```python
from build123d import *

# Parameters (mm, degrees)
BOSS_EXTRUDE1_DEPTH     = 4
CUT_EXTRUDE1_DEPTH      = 8.549834435
CUT_EXTRUDE1_DEPTH_BACK = 8.549834435
FILLET1_R               = 0.5
SKETCH4_R               = 1.5
BOSS_EXTRUDE2_DEPTH     = 1
SKETCH5_R               = 3.2
BOSS_EXTRUDE3_DEPTH     = 2.5
FILLET2_R               = 1
SKETCH6_W               = 1
SKETCH6_H               = 4.4
SKETCH6_W_2             = 4.4
SKETCH6_H_2             = 1
CUT_EXTRUDE_THIN1_DEPTH = 1.25
SKETCH8_W               = 7.4
SKETCH8_H               = 7.4
BOSS_EXTRUDE4_DEPTH     = 1


with BuildPart() as part:
    # Sketch1 → Boss-Extrude1 (new, symmetric)
    with BuildSketch(Plane.XY):
        with BuildLine():
            Line((-1.75, 1), (-1.75, -4.5))
            ThreePointArc((-1.75, -4.5), (-2.5, -5), (-3.25, -4.5))
            Line((-3.25, -4.5), (-3.25, 0))
            Line((-3.25, 0), (-4, 0))
            Line((-4, 0), (-4, 2.9))
            ThreePointArc((-4, 2.9), (-3.853553391, 3.253553391), (-3.5, 3.4))
            Line((-3.5, 3.4), (3.5, 3.4))
            ThreePointArc((3.5, 3.4), (3.853553391, 3.253553391), (4, 2.9))
            Line((4, 2.9), (4, 0))
            Line((4, 0), (3.25, 0))
            Line((3.25, 0), (3.25, -4.5))
            ThreePointArc((3.25, -4.5), (2.5, -5), (1.75, -4.5))
            Line((1.75, -4.5), (1.75, 1))
            Line((1.75, 1), (-1.75, 1))
        make_face()
    extrude(amount=BOSS_EXTRUDE1_DEPTH, both=True)

    # Sketch3 → Cut-Extrude1 (cut, two sides: drawn at the far end of the back side and taken through both)
    with BuildSketch(Plane(origin=(0, 0, 0), x_dir=(0, 0, -1), z_dir=(1, 0, 0)).offset(-CUT_EXTRUDE1_DEPTH_BACK)):
        with BuildLine():
            Line((-3.2, -5), (-3.2, 2.1))
            ThreePointArc((-3.2, 2.1), (-3.053553391, 2.453553391), (-2.7, 2.6))
            Line((-2.7, 2.6), (2.7, 2.6))
            ThreePointArc((2.7, 2.6), (3.053553391, 2.453553391), (3.2, 2.1))
            Line((3.2, 2.1), (3.2, -5))
            Line((3.2, -5), (-3.2, -5))
        make_face()
    extrude(amount=CUT_EXTRUDE1_DEPTH + CUT_EXTRUDE1_DEPTH_BACK, mode=Mode.SUBTRACT)

    # Fillet1
    # the kernel refuses this fillet: 0.5 mm, written as the material it takes off along each edge
    with BuildSketch(Plane(origin=(-4.75, 3.4, -4), x_dir=(0, -1, 0), z_dir=(1, 0, 0))) as fillet1_piece_1:
        with BuildLine():
            CenterArc((FILLET1_R, -FILLET1_R), FILLET1_R, 90, 90)
            Line((0, -FILLET1_R), (0, 0))
            Line((0, 0), (FILLET1_R, 0))
        make_face()
    extrude(amount=9.5, mode=Mode.SUBTRACT)
    with BuildSketch(Plane(origin=(-4.75, 3.4, 4), x_dir=(0, -1, 0), z_dir=(1, 0, 0))) as fillet1_piece_2:
        with BuildLine():
            CenterArc((FILLET1_R, FILLET1_R), FILLET1_R, 180, 90)
            Line((0, FILLET1_R), (0, 0))
            Line((0, 0), (FILLET1_R, 0))
        make_face()
    extrude(amount=9.5, mode=Mode.SUBTRACT)

    # Sketch4 → Boss-Extrude2 (add)
    with BuildSketch(Plane(origin=(0, 3.4, 0), x_dir=(1, 0, 0), z_dir=(0, 1, 0))):
        with Locations(Location((0, 0, 0), (0, 0, 90))):
            Circle(SKETCH4_R)
    extrude(amount=BOSS_EXTRUDE2_DEPTH)

    # Sketch5 → Boss-Extrude3 (add)
    with BuildSketch(Plane(origin=(0, 4.4, 0), x_dir=(1, 0, 0), z_dir=(0, 1, 0))):
        with Locations(Location((0, 0, 0), (0, 0, 270))):
            Circle(SKETCH5_R)
    extrude(amount=BOSS_EXTRUDE3_DEPTH)

    # Fillet2
    fillet2_edges = [part.edges().sort_by_distance(p)[0] for p in [
        (0, 4.4, -3.2),
        (0, 6.9, -3.2),
    ]]
    fillet(fillet2_edges, radius=FILLET2_R)

    # Sketch6 → Cut-Extrude-Thin1 (cut)
    with BuildSketch(Plane(origin=(0, 6.9, 0), x_dir=(1, 0, 0), z_dir=(0, 1, 0))):
        Rectangle(SKETCH6_W, SKETCH6_H)
        Rectangle(SKETCH6_W_2, SKETCH6_H_2)
    extrude(amount=-CUT_EXTRUDE_THIN1_DEPTH, mode=Mode.SUBTRACT)

    # Sketch8 → Boss-Extrude4 (add)
    with BuildSketch(Plane(origin=(0, 3.4, 0), x_dir=(1, 0, 0), z_dir=(0, 1, 0))):
        Rectangle(SKETCH8_W, SKETCH8_H)
    extrude(amount=BOSS_EXTRUDE4_DEPTH)


solid = part.part
```
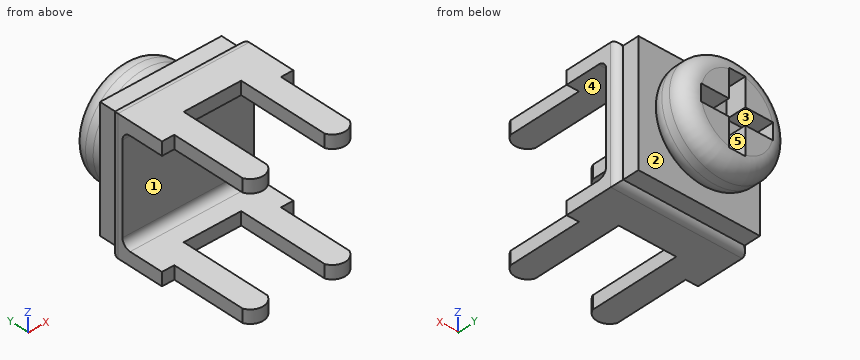
Work out the finished part from the listing and answer in its coordinate system (mm). Face numbers are marked on the shaded views. A direction names the side the tool comes from. Coordinates: 2 decimals unless noted, no trailing zeros. Loops run counter-clockwise (first coordinate to the right, second up) from the corner with the lowest first, then second, coordinate; pieces in that order, holes last. Notation, with made-up numbers: (-31.75, 79.5) - (-0.75, 79.5) arc R8 cw to (-0.75, 93.5) - close; hole circle Ø2 at (-9.75, 7). An arc over 180 degrees is marked (long way). Use a Markdown table: item, result.
Item 1: Consider probe 1 along Z at (x, y) = (-3, 0.5); probe 2 along X at (y, z) = (-1.5, -3.5); probe 3 along Y at (x, z) = (1.5, -0.25). Determine where each line is inside the solid, lowest interval first. Write a range as from..to.
Evaluation:
| item | result |
|---|---|
| probe 1 | z = -4..-3.2, 3.2..4 |
| probe 2 | x = -3.25..-1.75, 1.75..3.25 |
| probe 3 | y = 2.6..5.65 |
Item 2: The mould has two halves that part along X. Classify the marked faces 4 and 5: +X half, -X half, draft (parallel to the pull), parting line (faces both ways), or undercut.
Evaluation:
| item | result |
|---|---|
| face 4 | draft |
| face 5 | undercut |
Item 3: For the marked faces 1, 2 and 3, determine the directions among +Z, -Z, +X, -X, +Y, -Y from which every point of the face is accessible in a straight line to the end or side of a thin tool.
Evaluation:
| item | result |
|---|---|
| face 1 | +X, -X, -Y |
| face 2 | none |
| face 3 | +Y |
Item 4: Find section B-B, the plane z = 0. Determine the outline of the cut face in (x, y).
Evaluation:
| item | result |
|---|---|
| outline | (-4, 2.6) - (4, 2.6) - (4, 2.9) arc R0.5 ccw to (3.5, 3.4) - (3.7, 3.4) - (3.7, 4.4) - (2.2, 4.4) arc R1 ccw to (3.2, 5.4) - (3.2, 5.9) arc R1 ccw to (2.2, 6.9) - (2.2, 5.65) - (-2.2, 5.65) - (-2.2, 6.9) arc R1 ccw to (-3.2, 5.9) - (-3.2, 5.4) arc R1 ccw to (-2.2, 4.4) - (-3.7, 4.4) - (-3.7, 3.4) - (-3.5, 3.4) arc R0.5 ccw to (-4, 2.9) - close |
Item 5: Find section A-A, the plane y = -4. Determine the outline of the cut face in (x, z).
Evaluation:
| item | result |
|---|---|
| outline | (-3.25, -4) - (-1.75, -4) - (-1.75, -3.2) - (-3.25, -3.2) - close; (-3.25, 3.2) - (-1.75, 3.2) - (-1.75, 4) - (-3.25, 4) - close; (1.75, -4) - (3.25, -4) - (3.25, -3.2) - (1.75, -3.2) - close; (1.75, 3.2) - (3.25, 3.2) - (3.25, 4) - (1.75, 4) - close |
Item 6: Find section C-C, the plane x = 0. Determine the outline of the cut face in (y, z), and give its area (3 significant figures).
Evaluation:
| item | result |
|---|---|
| outline | (1, -4) - (2.9, -4) arc R0.5 ccw to (3.4, -3.5) - (3.4, -3.7) - (4.4, -3.7) - (4.4, -2.2) arc R1 ccw to (5.4, -3.2) - (5.9, -3.2) arc R1 ccw to (6.9, -2.2) - (5.65, -2.2) - (5.65, 2.2) - (6.9, 2.2) arc R1 ccw to (5.9, 3.2) - (5.4, 3.2) arc R1 ccw to (4.4, 2.2) - (4.4, 3.7) - (3.4, 3.7) - (3.4, 3.5) arc R0.5 ccw to (2.9, 4) - (1, 4) - (1, 3.2) - (2.1, 3.2) arc R0.5 cw to (2.6, 2.7) - (2.6, -2.7) arc R0.5 cw to (2.1, -3.2) - (1, -3.2) - close |
| area | 26.0 mm2 |
Item 7: Given pin 1 Ø4 at (x, z) = (-2, 2.5) entering from -Y; pin 2 Ø0.8 at (y, z) = (6.5, 0) entering from -X; pin 3 Ø3 at (x, z) = (-1.5, -1) entering from -Y; pin 4 Ø0.5 at (y, z) = (4, 1.5) entering from -X, each flat-ended and moving along its own axis, determine where each tip first touches the part or whether it passes through.
Evaluation:
| item | result |
|---|---|
| pin 1 | stops at y = -5 |
| pin 2 | stops at x = -3.18 |
| pin 3 | stops at y = 2.6 |
| pin 4 | stops at x = -3.7 |
